```python
from build123d import *

# Parameters (mm, degrees)
F0_R     = 6.35
F1_DEPTH = 16.002
F2_R     = 9.652
F5_DEPTH = 16.002
F6_R     = 9.652
F7_DEPTH = 57.151


with BuildPart() as f1:
    # F0 (on Front) → F1 (new body)
    with BuildSketch(Plane.XZ):
        with BuildLine():
            Line((-50.8, 0), (0, 0))
            Line((0, 0), (50.8, 0))
            Line((50.8, 0), (50.8, 44.45))
            ThreePointArc((50.8, 44.45), (38.1, 57.15), (25.4, 44.45))
            Line((25.4, 44.45), (25.4, 16.002))
            Line((25.4, 16.002), (0, 16.002))
            Line((0, 16.002), (-25.4, 16.002))
            Line((-25.4, 16.002), (-25.4, 44.45))
            ThreePointArc((-25.4, 44.45), (-38.1, 57.15), (-50.8, 44.45))
            Line((-50.8, 44.45), (-50.8, 0))
        make_face()
        with Locations((-38.1, 44.45)):
            Circle(F0_R, mode=Mode.SUBTRACT)
        with Locations((38.1, 44.45)):
            Circle(F0_R, mode=Mode.SUBTRACT)
    extrude(amount=F1_DEPTH)

    # F2
    f2_edges = [f1.edges().sort_by_distance(p)[0] for p in [
        (-25.4, -8.001, 16.002),
        (25.4, -8.001, 16.002),
    ]]
    fillet(f2_edges, radius=F2_R)

    # F3 (on Top) → F5 (join)
    with BuildSketch(Plane.XY):
        with BuildLine():
            Line((38.1, -16.002), (0, -16.002))
            Line((0, -16.002), (-38.1, -16.002))
            Line((-38.1, -16.002), (-38.1, -33.528))
            ThreePointArc((-38.1, -33.528), (-33.933887, -43.585887), (-23.876, -47.752))
            Line((-23.876, -47.752), (0, -47.752))
            Line((0, -47.752), (23.876, -47.752))
            ThreePointArc((23.876, -47.752), (33.933887, -43.585887), (38.1, -33.528))
            Line((38.1, -33.528), (38.1, -16.002))
        make_face()
    extrude(amount=F5_DEPTH)

    # F6
    f6_edges = [f1.edges().sort_by_distance(p)[0] for p in [
        (-38.1, -16.002, 8.001),
        (38.1, -16.002, 8.001),
    ]]
    fillet(f6_edges, radius=F6_R)

    # F4 (on Top) → F7 (cut, through all)
    with BuildSketch(Plane.XY):
        with BuildLine():
            Line((19.05, -25.4), (0, -25.4))
            Line((0, -25.4), (-19.05, -25.4))
            ThreePointArc((-19.05, -25.4), (-25.4, -31.75), (-19.05, -38.1))
            Line((-19.05, -38.1), (0, -38.1))
            Line((0, -38.1), (19.05, -38.1))
            ThreePointArc((19.05, -38.1), (25.4, -31.75), (19.05, -25.4))
        make_face()
    extrude(amount=F7_DEPTH, mode=Mode.SUBTRACT)


solid = f1.part
```
Work out the finished part from the listing and answer in its coordinate system (mm). A direction names the side the tool comes from. Give positions to 0.01 mm unless a question says otherwise; leave off trailing zeros. Loops run counter-clockwise (first coordinate to the right, second up) from the corner with the lowest first, then second, coordinate; pieces in that order, holes last. Notation, with made-up numbers: (76, 72) - (94, 72) arc R12 cw to (94, 81) - close; hole circle Ø5 at (-5.5, 51). An arc over 180 degrees is marked (long way). Use CSV: the item, a comma, the result in double quotes. Start each with the question number.
(1) Find the intervals of material crossed by L1, parallel to Z at x = -38, y = -7; L2, parallel to X at y = -14, z = 25.5; L3, parallel to Z at x = 0, y = -18.5, in increasing order.
(2) A tool of negligible diameter and unlimited length cuts with its end or side. For faces 5 (the face through (22.648, -8.113, 18.904)), 6 (the face through (-1, -24, 16.002)), 7 (the face through (-38.1, -30, 8)), 8 (the face through (-38.927, -7.889, 50.746)), 9 (the face through (-25.4, -31.6, 7.9)), from which of +Z, -Z, +X, -X, +Y, -Y can it reach the whole face along a straight path? Write none if from no direction.
(3) Each of these flat-tipped pins is pushed along its axis until it touches: pin 1 (4 mm diameter, centred on x = -5.5, y = -5, fed in from +Z); pin 2 (6.5 mm diameter, centred on y = -30.5, z = 6.5, fed in from +X); pin 3 (2.5 mm diameter, centred on y = -28, z = 10, fed in from -X). Where does it stop, or does it pass through?
(4) Find section C-C, the plane y = -14. Determine the outline of the cut face in (x, z).
(5) Find section A-A, the plane y = -31.75. Determine the outline of the cut face in (x, z).
(6) Determine the mould class of faces 1 (the face through (-22.648, -8.113, 18.904)), 2 (the face through (37, -16.002, 29)), 3 (the face through (-1, 0, 10)), 4 (the face through (25.4, -31.9, 7.9)) for opening direction Y: released by +Y, released by -Y, zero draft, split by the parting line, or undercut.
(7) Find section D-D, the plane x = 21. Determine the outline of the cut face in (y, z), plus the area to 3 significant figures.
(8) Find section B-B, the plane z = 52. Determine the outline of the cut face in (x, y).
Results found:
1,L1,"0 to 38.1, 50.8 to 57.15"
1,L2,"-50.8 to -25.4, 25.4 to 50.8"
1,L3,"0 to 16"
2,face 5,"+Z, +Y, -Y"
2,face 6,"+Z, -Y"
2,face 7,"+Z, -Z, -X, -Y"
2,face 8,"+Y, -Y"
2,face 9,"+Z, -Z"
3,pin 1,"z = 16"
3,pin 2,"x = 38.1"
3,pin 3,"x = -38.1"
4,outline,"(-50.8, 0) - (50.8, 0) - (50.8, 44.45) arc R12.7 ccw to (25.4, 44.45) - (25.4, 25.65) arc R9.65 cw to (15.75, 16) - (-15.75, 16) arc R9.65 cw to (-25.4, 25.65) - (-25.4, 44.45) arc R12.7 ccw to (-50.8, 44.45) - close; hole circle Ø12.7 at (-38.1, 44.45); hole circle Ø12.7 at (38.1, 44.45)"
5,outline,"(-38.1, 0) - (-25.4, 0) - (-25.4, 16) - (-38.1, 16) - close; (25.4, 0) - (38.1, 0) - (38.1, 16) - (25.4, 16) - close"
6,face 1,"zero draft"
6,face 2,"released by -Y"
6,face 3,"released by +Y"
6,face 4,"undercut"
7,outline,"(-47.75, 0) - (-37.79, 0) - (-37.79, 16) - (-47.75, 16) - close; (-25.71, 0) - (0, 0) - (0, 17.56) - (-16, 17.56) - (-16, 16) - (-25.71, 16) - close"
7,area,"596 mm^2"
8,outline,"(-48.31, -16) - (-27.89, -16) - (-27.89, 0) - (-48.31, 0) - close; (27.89, -16) - (48.31, -16) - (48.31, 0) - (27.89, 0) - close"
